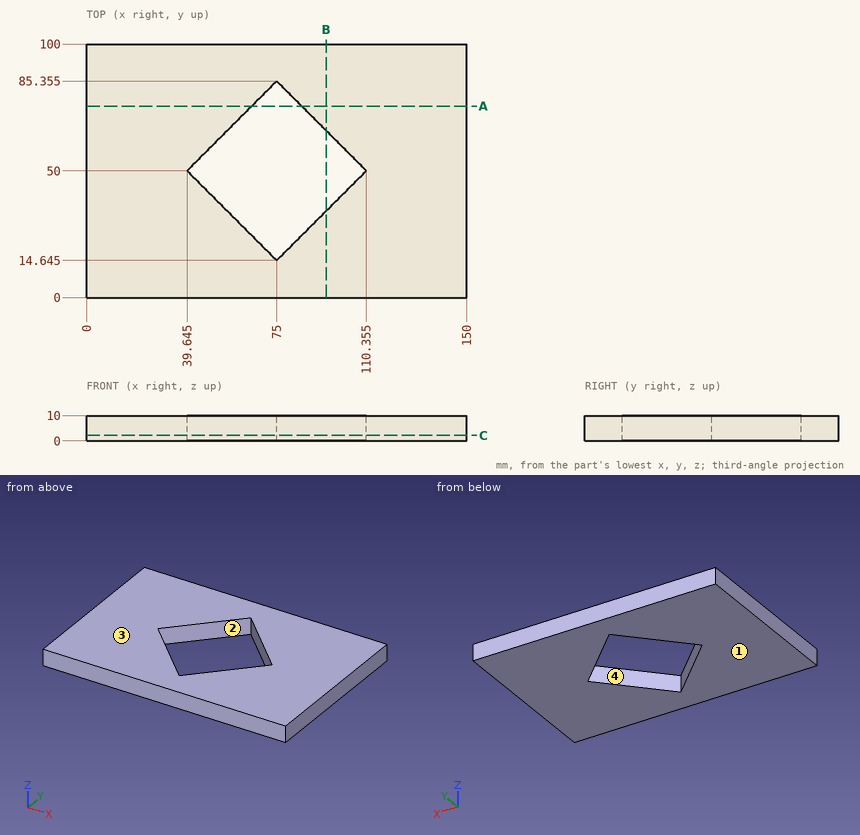
Answer from the drawing. Dimensions are ordinates in mm from the lowest x, y and z of the part. A direction names the side the tool comes from. Coordinates: 2 decimals unless noted, no trailing zeros. Order: outer loops, then holes, each group sorted by start corner. A loop starts at its lowest first (then second) coordinate and runs counter-clockwise, first axis right, second up. Notation, with made-up numbers: (86.5, 88.25) - (99.5, 88.25) arc R30 cw to (99.5, 123.25) - close; hole circle Ø4 at (-14.5, -16.75). An arc over 180 degrees is marked (long way). Use one line per item in the form item = value.
(1) Section A-A, the plane y = 75.5 is taken. Give the vertices of the cut face in (x, z) (1 decimal), then the cut area to 3 significant figures.
Computed values:
outline = (0, 0) - (65.1, 0) - (65.1, 10) - (0, 10) - close; (84.9, 0) - (150, 0) - (150, 10) - (84.9, 10) - close
area = 1,300 mm²
(2) Section B-B, the plane x = 94.5 is taken. Give the vertices of the cut face in (y, z) (1 decimal), then the cut area to 3 significant figures.
Computed values:
outline = (0, 0) - (34.1, 0) - (34.1, 10) - (0, 10) - close; (65.9, 0) - (100, 0) - (100, 10) - (65.9, 10) - close
area = 683 mm²
(3) For a pull along X with two mould halves and no side action, classify the marked faces 1 and 2 as pulls with the +X half, pulls with the -X half, needs draft (parallel to the pull), parting line crosses it, or undercut.
Computed values:
face_1 = needs draft
face_2 = undercut
(4) Which of the six approach directions +Z, -Z, +X, -X, +Y, -Y give full straight-line access (tool end or side, diameter ignored) to the marked faces 3 and 4?
Computed values:
face_3 = +Z, +X, -X, +Y, -Y
face_4 = +Z, -Z
(5) Straight lines are drawn through the part: L1, parallel to X at y = 77, z = 2 (1 decimal); L2, parallel to Y at x = 87, z = 3 (1 decimal); L3, parallel to X at y = 58.5, z = 2.5 (1 decimal). For each, find the intervals that lie inside material, in ascending order.
Computed values:
L1 = 0 to 66.6, 83.4 to 150
L2 = 0 to 26.6, 73.4 to 100
L3 = 0 to 48.1, 101.9 to 150
(6) Section C-C, the plane z = 2.25 is taken. Give the vertices of the cut face in (x, y) (1 decimal).
Computed values:
outline = (0, 0) - (150, 0) - (150, 100) - (0, 100) - close; hole (39.6, 50) - (75, 14.6) - (110.4, 50) - (75, 85.4) - close
